Verification items for the finished model (mm, model axes). Coordinates: 2 decimals unless noted, no trailing zeros. Order: outer loops, then holes, each group sorted by start corner. A loop starts at its lowest first (then second) coordinate and runs counter-clockwise, first axis right, second up. Notation, with made-up numbers: M 11,60 L 67,60 A21 cw 67,68 Z; hole C 86,57.5 d3. An arc over 180 degrees is marked long. Return JSON: item names as keys, results as strings. Group by question number.
Q1. Thickness scan on probe 1 along Y at (x, z) = (50, 8.75); probe 2 along Y at (x, z) = (20, 8.5) (3 decimals); probe 3 along Y at (x, z) = (33, 13). Record the ranges inside material, lowest first.
Q2. Section check A-A, the plane x = 50. Enter the section's corners in (y, z).
Q3. Go/stop test with flat-tipped pins: pin 1 Ø1.5 at (y, z) = (14.5, 7.5) entering from -X; pin 2 Ø3 at (x, y) = (40.5, 18.5) entering from +Z; pin 3 Ø8 at (x, z) = (67, 14) entering from -Y; pin 4 Ø2 at (x, z) = (48, 12) entering from +Y. Record where each tip stops, or that it passes through.
Q4. Section check C-C, the plane x = 70. Enter the section's corners in (y, z).
Q5. Section check D-D, the plane y = 27.75. Enter the section's corners in (x, z), then the cut area to 3 significant figures.
Q6. Section check B-B, the plane z = 19. Count the separate pieces of the cut face and the enclosed holes in it, then the cut area to 3 significant figures.
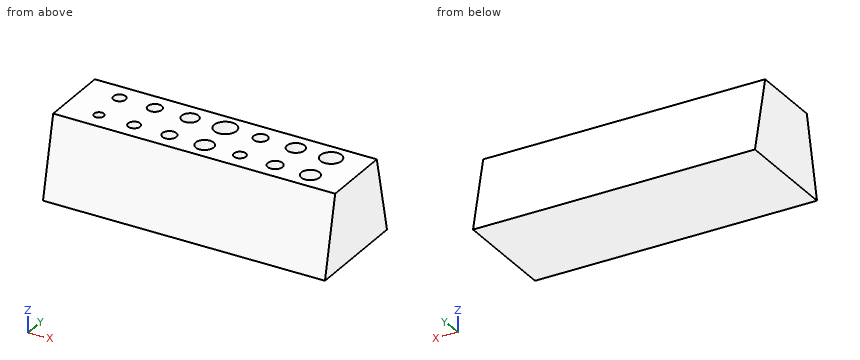
from build123d import *

# Parameters (mm, degrees)
F0_R     = 1.39
F0_R_2   = 1.725
F0_R_3   = 1.985
F0_R_4   = 2.55
F0_R_5   = 1.7
F0_R_6   = 2.1
F0_R_7   = 2.6
F0_R_8   = 1.75
F0_R_9   = 2.38
F0_R_10  = 3.175
F0_R_11  = 2
F0_R_12  = 2.5
F0_R_13  = 3
F1_DEPTH = 22
F2_DEPTH = 3
F4_DEPTH = 300


with BuildPart() as f1:
    # F0 (on Top) → F1 (new body)
    with BuildSketch(Plane.XY):
        Polygon((0, 30), (0, 0), (10, 0), (20, 0), (30, 0), (40, 0), (50, 0), (60, 0), (70, 0), (80, 0), (80, 30), align=None)
        with Locations((10, 10)):
            Circle(F0_R, mode=Mode.SUBTRACT)
        with Locations((20, 10)):
            Circle(F0_R_2, mode=Mode.SUBTRACT)
        with Locations((30, 10)):
            Circle(F0_R_3, mode=Mode.SUBTRACT)
        with Locations((40, 10)):
            Circle(F0_R_4, mode=Mode.SUBTRACT)
        with Locations((50, 10)):
            Circle(F0_R_5, mode=Mode.SUBTRACT)
        with Locations((60, 10)):
            Circle(F0_R_6, mode=Mode.SUBTRACT)
        with Locations((70, 10)):
            Circle(F0_R_7, mode=Mode.SUBTRACT)
        with Locations((10, 20)):
            Circle(F0_R_8, mode=Mode.SUBTRACT)
        with Locations((20, 20)):
            Circle(F0_R_3, mode=Mode.SUBTRACT)
        with Locations((30, 20)):
            Circle(F0_R_9, mode=Mode.SUBTRACT)
        with Locations((40, 20)):
            Circle(F0_R_10, mode=Mode.SUBTRACT)
        with Locations((50, 20)):
            Circle(F0_R_11, mode=Mode.SUBTRACT)
        with Locations((60, 20)):
            Circle(F0_R_12, mode=Mode.SUBTRACT)
        with Locations((70, 20)):
            Circle(F0_R_13, mode=Mode.SUBTRACT)
    extrude(amount=F1_DEPTH)

    # F0 (on Top) → F2 (join)
    with BuildSketch(Plane.XY):
        with Locations((70, 20)):
            Circle(F0_R_13)
        with Locations((70, 10)):
            Circle(F0_R_7)
        with Locations((60, 10)):
            Circle(F0_R_6)
        with Locations((60, 20)):
            Circle(F0_R_12)
        with Locations((50, 20)):
            Circle(F0_R_11)
        with Locations((50, 10)):
            Circle(F0_R_5)
        with Locations((40, 20)):
            Circle(F0_R_10)
        with Locations((40, 10)):
            Circle(F0_R_4)
        with Locations((30, 10)):
            Circle(F0_R_3)
        with Locations((30, 20)):
            Circle(F0_R_9)
        with Locations((20, 20)):
            Circle(F0_R_3)
        with Locations((20, 10)):
            Circle(F0_R_2)
        with Locations((10, 20)):
            Circle(F0_R_8)
        with Locations((10, 10)):
            Circle(F0_R)
    extrude(amount=F2_DEPTH)

    # F3 (on face) → F4 (cut)
    with BuildSketch(Plane(origin=(0, 0, 0), x_dir=(0, -1, 0), z_dir=(-1, 0, 0))):
        Polygon((-30, 22), (-30, 0), (-25.067758, 22), align=None)
        Polygon((-4.932242, 22), (0, 0), (0, 22), align=None)
    extrude(amount=-F4_DEPTH, mode=Mode.SUBTRACT)


solid = f1.part
Numbers:
{
 "1": {"probe 1": "y = 1.96 to 8.3, 11.7 to 18, 22 to 28.04", "probe 2": "y = 1.906 to 8.275, 11.725 to 18.015, 21.985 to 28.094", "probe 3": "y = 2.91 to 27.09"},
 "2": {"outline": "M 0,0 L 30,0 L 25.07,22 L 22,22 L 22,3 L 18,3 L 18,22 L 11.7,22 L 11.7,3 L 8.3,3 L 8.3,22 L 4.93,22 Z"},
 "3": {"pin 1": "stops at x = 0", "pin 2": "stops at z = 3", "pin 3": "stops at y = 2.24", "pin 4": "stops at y = 27.53"},
 "4": {"outline": "M 0,0 L 30,0 L 25.07,22 L 23,22 L 23,3 L 17,3 L 17,22 L 12.6,22 L 12.6,3 L 7.4,3 L 7.4,22 L 4.93,22 Z"},
 "5": {"outline": "M 0,0 L 80,0 L 80,10.04 L 0,10.04 Z", "area": "803 mm2"},
 "6": {"separate pieces": "1", "enclosed holes": "14", "area": "1,490 mm2"}
}
